Build history of the part. All positions in model axes, mm. Round coordinates to 2 decimals unless told otherwise and drop trailing zeros. Loops run counter-clockwise (first coordinate to the right, second up) from the corner with the lowest first, then second, coordinate; pieces in that order, holes last. Notation, with made-up numbers: (19, 38.25) - (56, 38.25) arc R25 ccw to (56, 75.25) - close; hole circle Ø11 at (-9, 74). An arc over 180 degrees is marked (long way). Use a Markdown table: item, result.
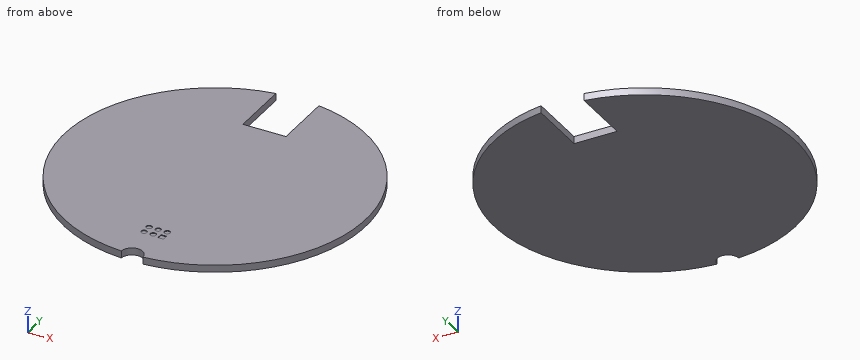
from build123d import *

# Parameters (mm, degrees)
F1_DEPTH = 1
F3_R     = 0.4
F3_W     = 0.8
F3_H     = 0.8
F4_DEPTH = 0.1


with BuildPart() as f1:
    # F0 (on Top) → F1 (new body)
    with BuildSketch(Plane.XY):
        with BuildLine():
            ThreePointArc((-1.499043, -20.946429), (0, -19.5), (1.499043, -20.946429))
            ThreePointArc((1.499043, -20.946429), (20.98643, -0.754827), (3, 20.78461))
            Line((3, 20.78461), (3, 12.45))
            Line((3, 12.45), (-3, 12.45))
            Line((-3, 12.45), (-3, 20.78461))
            ThreePointArc((-3, 20.78461), (-20.98643, -0.754827), (-1.499043, -20.946429))
        make_face()
    extrude(amount=F1_DEPTH)

    # F3 (on face) → F4 (cut)
    with BuildSketch(Plane.XY.offset(1)):
        with Locations((0, -15.62)):
            Circle(F3_R)
        with Locations((-1.27, -15.62)):
            Circle(F3_R)
        with Locations((1.27, -14.35)):
            Circle(F3_R)
        with Locations((0, -14.35)):
            Circle(F3_R)
        with Locations((-1.27, -14.35)):
            Circle(F3_R)
        with Locations((1.27, -15.62)):
            Rectangle(F3_W, F3_H)
    extrude(amount=-F4_DEPTH, mode=Mode.SUBTRACT)


solid = f1.part
Q1. Cut at C-C, the plane y = -11.5. List the corners of the cut face in (x, z).
Results found:
| item | result |
|---|---|
| outline | (-17.57, 0) - (17.57, 0) - (17.57, 1) - (-17.57, 1) - close |
Q2. Cut at B-B, the plane z = 0.6. List the corners of the cut face in (x, y).
Results found:
| item | result |
|---|---|
| outline | (-3, 12.45) - (-3, 20.78) arc R21 ccw to (-1.5, -20.95) arc R1.5 cw to (1.5, -20.95) arc R21 ccw to (3, 20.78) - (3, 12.45) - close |
Q3. Cut at A-A, the plane y = 14.5. List the corners of the cut face in (x, z).
Results found:
| item | result |
|---|---|
| outline | (-15.19, 0) - (-3, 0) - (-3, 1) - (-15.19, 1) - close; (3, 0) - (15.19, 0) - (15.19, 1) - (3, 1) - close |
Q4. Cut at D-D, the plane x = -7. List the corners of the cut face in (y, z).
Results found:
| item | result |
|---|---|
| outline | (-19.8, 0) - (19.8, 0) - (19.8, 1) - (-19.8, 1) - close |
Q5. Probe line 1 (Y direction, x = -1.27, z = 0.95); line 2 (X direction, y = 12.5, z = 0.65); line 3 (X direction, y = 0.5, z = 0.15). List the from-to ranges inside material, lowest first.
Results found:
| item | result |
|---|---|
| line 1 | y = -20.2 to -16.02, -15.22 to -14.75, -13.95 to 12.45 |
| line 2 | x = -16.87 to -3, 3 to 16.87 |
| line 3 | x = -20.99 to 20.99 |
